Design review of the part built by this model. Coordinates are the model's own, in mm. A direction names the side the tool comes from. Coordinates: 2 decimals unless noted, no trailing zeros. Order: outer loops, then holes, each group sorted by start corner. A loop starts at its lowest first (then second) coordinate and runs counter-clockwise, first axis right, second up. Notation, with made-up numbers: (-5, -4.75) -> (35, -4.75) arc R8 ccw to (35, 0.25) -> close; hole circle Ø8 at (-28.75, -32). An arc over 180 degrees is marked (long way). Write item = value, one per line.
```python
from build123d import *

# Parameters (mm, degrees)
SKICA1_R                     = 7
P_IDAT_VYSUNUT_M1_DEPTH      = 103
SKICA2_W                     = 5
SKICA2_H                     = 2.75
ZKOSEN_1_SIZE                = 0.5
P_IDAT_VYSUNUT_M2_DEPTH      = 2
P_IDAT_VYSUNUT_M2_DEPTH_BACK = 2


with BuildPart() as part:
    # Skica1 → P_idat vysunut_m1 (new body)
    with BuildSketch(Plane.XY):
        Circle(SKICA1_R)
    extrude(amount=P_IDAT_VYSUNUT_M1_DEPTH)

    # Skica2 → Rotovat1 (revolve)
    with BuildSketch(Plane(origin=(0, 0, 0), x_dir=(1, 0, 0), z_dir=(0, 1, 0)), mode=Mode.PRIVATE) as rotovat1_sk:
        with Locations((7.5, -31.875)):
            Rectangle(SKICA2_W, SKICA2_H)
    revolve(rotovat1_sk.sketch.rotate(Axis((0, 0, 0), (0, 0, 1)), 180), axis=Axis((0, 0, 0), (0, 0, 1)))

    # Zkosen_1
    zkosen_1_edges = [part.edges().sort_by_distance(p)[0] for p in [
        (-7, 0, 0),
        (10, 0, 33.25),
        (10, 0, 30.5),
        (-7, 0, 103),
    ]]
    chamfer(zkosen_1_edges, length=ZKOSEN_1_SIZE)

    # Skica5 → P_idat vysunut_m2 (add, two sides: drawn at the far end of the back side and taken through both)
    with BuildSketch(Plane(origin=(0, 7, 0), x_dir=(1, 0, 0), z_dir=(0, 1, 0)).offset(-P_IDAT_VYSUNUT_M2_DEPTH_BACK)):
        with BuildLine():
            Line((2.5, -80.5), (2.5, -95.5))
            ThreePointArc((2.5, -95.5), (0, -98), (-2.5, -95.5))
            Line((-2.5, -95.5), (-2.5, -80.5))
            ThreePointArc((-2.5, -80.5), (0, -78), (2.5, -80.5))
        make_face()
    extrude(amount=P_IDAT_VYSUNUT_M2_DEPTH + P_IDAT_VYSUNUT_M2_DEPTH_BACK)


solid = part.part
```
(1) For L1, parallel to Z at x = 7, y = 2.5; L2, parallel to Y at x = 0, z = 59; L3, parallel to X at y = 6.5, z = 70, list the stretches that pass through material, from the lowest coordinate up.
Report:
L1 = 30.5 to 33.25
L2 = -7 to 7
L3 = -2.6 to 2.6
(2) Insertion check: pin 1 (1.2 mm diameter, centred on y = 7, z = 91, fed in from -X); pin 2 (2 mm diameter, centred on y = 8, z = 88, fed in from +X); pin 3 (1.5 mm diameter, centred on y = 3, z = 89, fed in from -X); pin 4 (8 mm diameter, centred on x = 7, y = 7, fed in from +Z). Each pin has a flat end and moves straight along its axis. Give the tip position at first contact, or say it passes through.
Report:
pin_1 = -2.84
pin_2 = 2.5
pin_3 = -6.63
pin_4 = 103
(3) We need section A-A (x = 0). Write out the cut boundary in (y, z), and give its area (3 significant figures).
Report:
outline = (-10, 31) -> (-9.5, 30.5) -> (-7, 30.5) -> (-7, 0.5) -> (-6.5, 0) -> (6.5, 0) -> (7, 0.5) -> (7, 30.5) -> (9.5, 30.5) -> (10, 31) -> (10, 32.75) -> (9.5, 33.25) -> (7, 33.25) -> (7, 78) -> (9, 78) -> (9, 98) -> (7, 98) -> (7, 102.5) -> (6.5, 103) -> (-6.5, 103) -> (-7, 102.5) -> (-7, 33.25) -> (-9.5, 33.25) -> (-10, 32.75) -> close
area = 1,500 mm²
(4) The part is to be moulded in two halves that separate along Z. For faces 4 (the cylindrical face through (10, 0, 32)), 5 (the cylindrical face through (0, 8, 78)), 6 (the cylindrical face through (0, 8, 98)), 7 (the flat face through (0, 0, 0)), say which applies: released by +Z, released by -Z, zero draft, split by the parting line, or undercut.
Report:
face_4 = zero draft
face_5 = undercut
face_6 = released by +Z
face_7 = released by -Z
(5) We need section B-B (y = 0). Write out the cut boundary in (x, z).
Report:
outline = (-10, 31) -> (-9.5, 30.5) -> (-7, 30.5) -> (-7, 0.5) -> (-6.5, 0) -> (6.5, 0) -> (7, 0.5) -> (7, 30.5) -> (9.5, 30.5) -> (10, 31) -> (10, 32.75) -> (9.5, 33.25) -> (7, 33.25) -> (7, 102.5) -> (6.5, 103) -> (-6.5, 103) -> (-7, 102.5) -> (-7, 33.25) -> (-9.5, 33.25) -> (-10, 32.75) -> close
(6) For faces 1 (the flat face through (-2.5, 8, 88)), 2 (the flat face through (-4, 6, 30.5)), 3 (the flat face through (2.5, 8, 88)), list the 3-axis set-ups (+Z, -Z, +X, -X, +Y, -Y) from which the entire face can be reached by the end or side of a thin tool; tool diameter is ignored.
Report:
face_1 = +Z, -X, +Y
face_2 = -Z
face_3 = +Z, +X, +Y
(7) We need section C-C (z = 22). Write out the cut boundary in (x, y).
Report:
outline = circle Ø14 at (0, 0)
